Read the model definition and answer for the solid it produces. Units are mm, in the model's axes. A direction names the side the tool comes from. Give positions to 0.01 mm unless a question says otherwise; leave off trailing zeros. Loops run counter-clockwise (first coordinate to the right, second up) from the corner with the lowest first, then second, coordinate; pieces in that order, holes last. Notation, with made-up numbers: (-19.5, -22.5) - (6.5, -22.5) arc R22 ccw to (6.5, -2.5) - close; hole circle Ø3 at (-19, 75.25). An arc over 180 degrees is marked (long way). Write each question's results on one line, items separated by ' | '. Start each with the question number.
Q1. The part is cut by section B-B, the plane y = 20. Write down the section's boundary in (x, z).
Q2. The part is cut by section C-C, the plane z = 22. Write down the section's boundary in (x, y), plus the area to 3 significant figures.
Q3. For faces 5 (the cylindrical face through (32.923, 33.226, 1.479)), 6 (the flat face through (-1, 26.5, 27)), 7 (the flat face through (21, 20, 3)), determine the directions among +Z, -Z, +X, -X, +Y, -Y from which every point of the face is accessible in a straight line to the end or side of a thin tool.
Q4. The part is cut by section D-D, the plane y = 12.25. Write down the section's boundary in (x, z), plus the area to 3 significant figures.
Q5. Determine the mould class of faces 1 (the cylindrical face through (-2.1, 20.28, 0.86)), 2 (the cylindrical face through (-1.48, 4.57, 25.5)), 3 (the cylindrical face through (-1.479, 12.701, 41.854)), 4 (the flat face through (9, 40, 2)) for opening direction Y: +Y half, -Y half, draft (parallel to the pull), parting line (faces both ways), or undercut.
Q6. Find the intervals of material crossed by line 1 (Y direction, x = 8, z = 2.2); line 2 (Y direction, x = -2, z = 27); line 3 (Z direction, x = -1, y = 27) (3 decimals), in increasing order. Write a range as from..to.
Q7. The part is cut by section A-A, the plane x = 32. Write down the section's boundary in (y, z).
Q8. Given pin 1 (2.5 mm diameter, centred on y = 35.5, z = 27, fed in from -X); pin 2 (5 mm diameter, centred on y = 12.25, z = 40.42, fed in from +X); pin 3 (11 mm diameter, centred on x = 28, y = 10.5, fed in from +Z), each flat-ended and moving along its own axis, determine where each tip first touches the part or whether it passes through.
```python
from build123d import *

# Parameters (mm, degrees)
SKETCH_1_W      = 40
SKETCH_1_H      = 40
SKETCH_1_R      = 2
EXTRUDE_1_DEPTH = 3
FILLET_1_R      = 5
SKETCH_2_R      = 1.5
EXTRUDE_2_DEPTH = 3
FILLET_2_R      = 3


with BuildPart() as part:
    # 草图1 → 凸台-拉伸1 (new body)
    with BuildSketch(Plane.XY):
        with Locations((20, 20)):
            Rectangle(SKETCH_1_W, SKETCH_1_H)
        with Locations((8, 35)):
            Circle(SKETCH_1_R, mode=Mode.SUBTRACT)
        with Locations((32, 35)):
            Circle(SKETCH_1_R, mode=Mode.SUBTRACT)
        with Locations((32, 5)):
            Circle(SKETCH_1_R, mode=Mode.SUBTRACT)
        with Locations((8, 5)):
            Circle(SKETCH_1_R, mode=Mode.SUBTRACT)
    extrude(amount=EXTRUDE_1_DEPTH)

    # 圆角1
    fillet_1_edges = [part.edges().sort_by_distance(p)[0] for p in [
        (40, 40, 1.5),
        (40, 0, 1.5),
    ]]
    fillet(fillet_1_edges, radius=FILLET_1_R)

    # 草图2 → 凸台-拉伸2 (add)
    with BuildSketch(Plane.ZY):
        with BuildLine():
            Line((0, 40), (27, 40))
            ThreePointArc((27, 40), (47, 20), (27, 0))
            Line((27, 0), (0, 0))
            Line((0, 0), (0, 40))
        make_face()
        with Locations((27, 35.5)):
            Circle(SKETCH_2_R, mode=Mode.SUBTRACT)
        with Locations((40.423393759, 27.75)):
            Circle(SKETCH_2_R, mode=Mode.SUBTRACT)
        with Locations((40.423393759, 12.25)):
            Circle(SKETCH_2_R, mode=Mode.SUBTRACT)
        with Locations((27, 4.5)):
            Circle(SKETCH_2_R, mode=Mode.SUBTRACT)
        with Locations((13.576606241, 12.25)):
            Circle(SKETCH_2_R, mode=Mode.SUBTRACT)
        with Locations((13.576606241, 27.75)):
            Circle(SKETCH_2_R, mode=Mode.SUBTRACT)
        with BuildLine():
            Line((20, 26.5), (34, 26.5))
            ThreePointArc((34, 26.5), (40.5, 20), (34, 13.5))
            Line((34, 13.5), (20, 13.5))
            ThreePointArc((20, 13.5), (13.5, 20), (20, 26.5))
        make_face(mode=Mode.SUBTRACT)
    extrude(amount=EXTRUDE_2_DEPTH)

    # 圆角2
    fillet_2_edges = [part.edges().sort_by_distance(p)[0] for p in [
        (-3, 20, 0),
        (0, 20, 3),
    ]]
    fillet(fillet_2_edges, radius=FILLET_2_R)


solid = part.part
```
Check sheet entries:
1) outline: (-3, 3) arc R3 ccw to (0, 0) - (40, 0) - (40, 3) - (3, 3) arc R3 cw to (0, 6) - (0, 13.5) - (-3, 13.5) - close; (-3, 40.5) - (0, 40.5) - (0, 47) - (-3, 47) - close
2) outline: (-3, 0) - (0, 0) - (0, 13.5) - (-3, 13.5) - close; (-3, 26.5) - (0, 26.5) - (0, 40) - (-3, 40) - close | area: 81.0 mm^2
3) face 5: +Z, -Z | face 6: +X, -X | face 7: +Z, +X, +Y, -Y
4) outline: (-3, 3) arc R3 ccw to (0, 0) - (40, 0) - (40, 3) - (3, 3) arc R3 cw to (0, 6) - (0, 12.08) - (-3, 12.08) - close; (-3, 15.08) - (0, 15.08) - (0, 38.92) - (-3, 38.92) - close; (-3, 41.92) - (0, 41.92) - (0, 45.44) - (-3, 45.44) - close | area: 238 mm^2
5) face 1: draft | face 2: undercut | face 3: undercut | face 4: +Y half
6) line 1: y = 0..3, 7..33, 37..40 | line 2: y = 0..3, 6..13.5, 26.5..34, 37..40 | line 3: z = 0.172..12.278, 14.876..39.124, 41.722..45.735
7) outline: (0, 0) - (3, 0) - (3, 3) - (0, 3) - close; (7, 0) - (33, 0) - (33, 3) - (7, 3) - close; (37, 0) - (40, 0) - (40, 3) - (37, 3) - close
8) pin 1: passes through | pin 2: stops at x = 0 | pin 3: stops at z = 3
